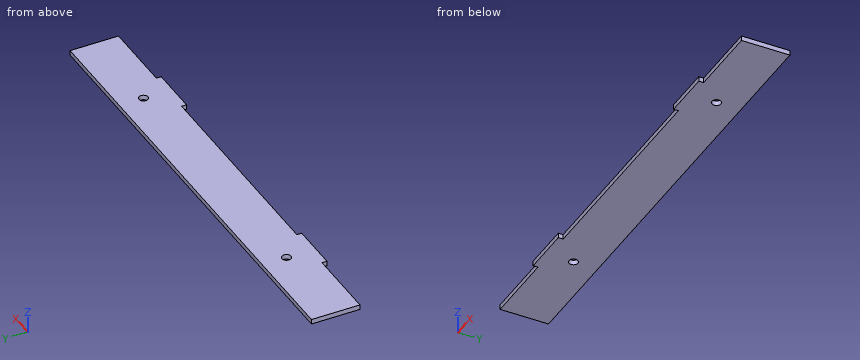
from build123d import *

# Parameters (mm, degrees)
SALIENTE_EXTRUIR1_DEPTH      = 1.5
TALADRO_DE_MARGEN_PARA_M51_D = 5.5


with BuildPart() as part:
    # Croquis1 → Saliente-Extruir1 (new, symmetric)
    with BuildSketch(Plane.XY):
        Polygon((-143.5, -15), (-98.5, -15), (-98.5, -18), (-68.5, -18), (-68.5, -15), (68.5, -15), (68.5, -18), (98.5, -18), (98.5, -15), (143.5, -15), (143.5, 15), (-143.5, 15), align=None)
    extrude(amount=SALIENTE_EXTRUIR1_DEPTH, both=True)

    # Taladro de margen para M51 (through all)
    with Locations(Plane.XY.offset(1.5)):
        with Locations((-85, 0), (85, 0)):
            Hole(TALADRO_DE_MARGEN_PARA_M51_D / 2)


solid = part.part
Part model, mm, in its own coordinate system. Give positions to 0.01 mm unless a question says otherwise; leave off trailing zeros. Loops run counter-clockwise (first coordinate to the right, second up) from the corner with the lowest first, then second, coordinate; pieces in that order, holes last. Notation, with made-up numbers: M 21.5,21.5 L 58.5,21.5 A21 ccw 58.5,32.5 Z; hole C 6,85 d4. An arc over 180 degrees is marked long. Put each result on its own line as item: value. Start each with the question number.
1) Saw through at A-A (z = -0.35). List the corners of the cut face in (x, y).
2) Saw through at D-D (x = 8.5). List the corners of the cut face in (y, z).
3) Flat gauge pins, fed straight in: pin 1 (0.9 mm diameter, centred on y = -16.5, z = -0.5, fed in from -X); pin 2 (0.9 mm diameter, centred on x = 122.5, z = 0.5, fed in from -Y); pin 3 (0.9 mm diameter, centred on y = -16.5, z = -0.5, fed in from +X). Where does each tip first touch, or does it go through?
4) Saw through at C-C (x = 85). List the corners of the cut face in (y, z), then the cut area to 3 significant figures.
5) Probe probe 1 along X at (y, z) = (-0.5, 0.65); probe 2 along Y at (x, z) = (85, 0.2); probe 3 along Y at (x, z) = (-67.5, 1). List the from-to ranges inside material, lowest first.
6) Saw through at B-B (y = 0). List the corners of the cut face in (x, z).
Numbers:
1. outline: M -143.5,-15 L -98.5,-15 L -98.5,-18 L -68.5,-18 L -68.5,-15 L 68.5,-15 L 68.5,-18 L 98.5,-18 L 98.5,-15 L 143.5,-15 L 143.5,15 L -143.5,15 Z; hole C -85,0 d5.5; hole C 85,0 d5.5
2. outline: M -15,-1.5 L 15,-1.5 L 15,1.5 L -15,1.5 Z
3. pin 1: x = -98.5
3. pin 2: y = -15
3. pin 3: x = 98.5
4. outline: M -18,-1.5 L -2.75,-1.5 L -2.75,1.5 L -18,1.5 Z; M 2.75,-1.5 L 15,-1.5 L 15,1.5 L 2.75,1.5 Z
4. area: 82.5 mm^2
5. probe 1: -143.5 to -87.7, -82.3 to 82.3, 87.7 to 143.5
5. probe 2: -18 to -2.75, 2.75 to 15
5. probe 3: -15 to 15
6. outline: M -143.5,-1.5 L -87.75,-1.5 L -87.75,1.5 L -143.5,1.5 Z; M -82.25,-1.5 L 82.25,-1.5 L 82.25,1.5 L -82.25,1.5 Z; M 87.75,-1.5 L 143.5,-1.5 L 143.5,1.5 L 87.75,1.5 Z
